```python
from build123d import *

# Parameters (mm, degrees)
SKETCH1_R           = 215.9
BOSS_EXTRUDE1_DEPTH = 88.9
BOSS_EXTRUDE1_TAPER = 20
BOSS_EXTRUDE2_DEPTH = 19.05
CIRPATTERN1_COUNT   = 2
SKETCH3_R           = 281.208754883
SKETCH3_R_2         = 280.708754883
EXTRUDE_THIN1_DEPTH = 1


with BuildPart() as part:
    # Sketch1 → Boss-Extrude1 (new body)
    with BuildSketch(Plane(origin=(0, 0, 0), x_dir=(1, 0, 0), z_dir=(0, 1, 0))):
        Circle(SKETCH1_R)
    extrude(amount=BOSS_EXTRUDE1_DEPTH, taper=BOSS_EXTRUDE1_TAPER)

    # Sketch2 → Boss-Extrude2 (add)
    with BuildSketch(Plane.XZ):
        with BuildLine():
            Line((-215.83125921, -5.447710344), (-200.854021104, -79.186313252))
            ThreePointArc((-200.854021104, -79.186313252), (-262.820614641, -40.008016754), (-278.934374009, 31.512220871))
            ThreePointArc((-278.934374009, 31.512220871), (-251.385968328, 6.197520074), (-215.83125921, -5.447710344))
        make_face()
    boss_extrude2 = extrude(amount=-BOSS_EXTRUDE2_DEPTH)

    # CirPattern1: Boss-Extrude2 ×2 about axis
    cirpattern1_axis = Axis((0, 0, 0), (0, 1, 0))
    for i in range(1, CIRPATTERN1_COUNT):
        add(boss_extrude2.rotate(cirpattern1_axis, i * 360 / CIRPATTERN1_COUNT))

    # Sketch3 → Extrude-Thin1 (add)
    with BuildSketch(Plane.XZ):
        Circle(SKETCH3_R)
        Circle(SKETCH3_R_2, mode=Mode.SUBTRACT)
    extrude(amount=-EXTRUDE_THIN1_DEPTH)


solid = part.part
```
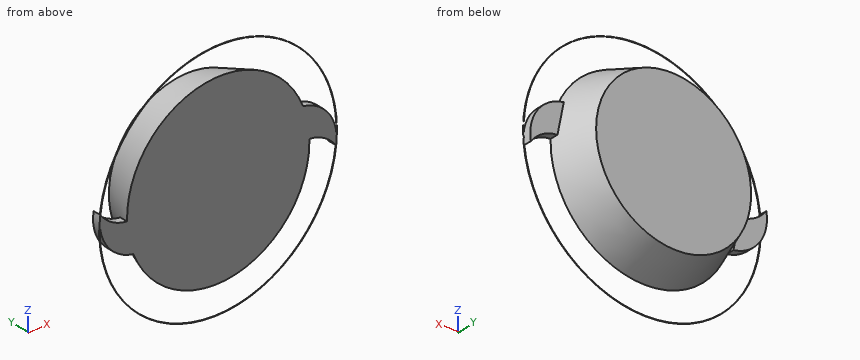
Geometry: final body of the model. Coordinates: model frame, mm. Round coordinates to 2 decimals unless told otherwise and drop trailing zeros. Order: outer loops, then holes, each group sorted by start corner. A loop starts at its lowest first (then second) coordinate and runs counter-clockwise, first axis right, second up. Notation, with made-up numbers: (61, -40) - (88, -40) arc R17 cw to (88, -12) - close; hole circle Ø9 at (55.5, 74.25). An arc over 180 degrees is marked (long way). Use CSV: the item, a comma, the result in double quotes. Start each with the question number.
Q1. Section query B-B (z = 244). Return loops of the section in (x, y).
Q2. Section query D-D (y = 36). Return loops of the section in (x, z).
Q3. Material intervals for line 1 along Z through (x, y) = (-97.5, 36.5); line 2 along Z through (x, y) = (-86, 43); line 3 along X through (y, z) = (13, -135), sorted ascending. Write a range as from..to.
Q4. First-contact query: pin 1 (6 mm diameter, centred on x = 161, y = 34, fed in from +Z); pin 2 (10 mm diameter, centred on x = -95, z = -145, fed in from -Y); pin 3 (1 mm diameter, centred on x = -150, y = 22.5, fed in from +Z); pin 4 (5 mm diameter, centred on x = 160, y = 38, fed in from -Z). Flat tips, straight axial feed; report the tip coordinate or a pass-through.
Q5. Section query C-C (z = -152). State how many separate pieces and enclosed holes the cut face has, and give its area (3 significant figures).
Q6. Section query A-A (x = 0). Return loops of the section in (y, z), and give its area (3 significant figures).
Result set:
1,outline,"(-139.79, 0) - (-138.79, 0) - (-138.79, 1) - (-139.79, 1) - close; (138.79, 0) - (139.79, 0) - (139.79, 1) - (138.79, 1) - close"
2,outline,"circle Ø405.59 at (0, 0)"
3,line 1,"z = -177.61..177.61"
3,line 2,"z = -180.84..180.84"
3,line 3,"x = -162.38..162.38"
4,pin 1,"stops at z = 128.68"
4,pin 2,"stops at y = 0"
4,pin 3,"stops at z = 144.26"
4,pin 4,"stops at z = -126.91"
5,separate pieces,"3"
5,enclosed holes,"0"
5,area,"23,000 mm2"
6,outline,"(0, -281.21) - (1, -281.21) - (1, -280.71) - (0, -280.71) - close; (0, -215.9) - (88.9, -183.54) - (88.9, 183.54) - (0, 215.9) - close; (0, 280.71) - (1, 280.71) - (1, 281.21) - (0, 281.21) - close"
6,area,"35,500 mm2"
